The listing builds one solid part. Answer for the finished solid, in the listing's coordinates (mm). Face numbers are marked on the shaded views. A direction names the side the tool comes from. Give positions to 0.01 mm unless a question says otherwise; leave off trailing zeros. Loops run counter-clockwise (first coordinate to the right, second up) from the corner with the lowest first, then second, coordinate; pieces in that order, holes last. Notation, with made-up numbers: (-14, 51) - (14, 51) arc R4 cw to (14, 56) - close; hole circle Ø7 at (1, 0.5). An arc over 180 degrees is marked (long way). Write each question's results on one line, items separated by ' | '.
Autodesk Inventor part; units mm, degrees
ref_plane "YZ Plane" through (0, 0, 0) normal (1, 0, 0) x (0, 1, 0)
ref_plane "XZ Plane" through (0, 0, 0) normal (0, 1, 0) x (-1, 0, 0)
ref_plane "XY Plane" through (0, 0, 0) normal (0, 0, 1) x (1, 0, 0)
sketch "Sketch1" plane through (0, 0, 0) normal (1, 0, 0) x (0, 1, 0)
  line L0 (0, 0) -> (230.2002, 0)
  line L1 (230.2002, 0) -> (230.2002, -138.176)
  line L2 (230.2002, -138.176) -> (0, -138.176)
  line L3 (0, -138.176) -> (0, 0)
  dimension "d0" = 230.2002
  dimension "d1" = 138.176
extrude "Extrusion1" add sketch "Sketch1" along normal blind 266.7
sketch "Sketch2" plane through (266.7, 0, 0) normal (1, 0, 0) x (0, 0, -1)
  line L0 (0, 230.2002) -> (0, 0)
  line L1 (0, 0) -> (138.176, 0)
  line L2 (138.176, 0) -> (138.176, 230.2002)
  line L3 (138.176, 230.2002) -> (0, 230.2002)
  line L4 (19.05, 211.1502) -> (63.5, 211.1502)
  line L5 (63.5, 211.1502) -> (63.5, 19.05)
  line L6 (63.5, 19.05) -> (19.05, 19.05)
  line L7 (19.05, 19.05) -> (19.05, 211.1502)
  dimension "d4" = 19.05
  dimension "d5" = 63.5
  dimension "d7" = 19.05
  dimension "d17" = 19.05
extrude "Extrusion2" cut sketch "Sketch2" against normal blind 266.7 contours L4 L5 L6 L7
sketch "Sketch3" plane through (0, 0, 0) normal (-1, 0, 0) x (0, 0, 1)
  line L0 (-19.05, 211.1502) -> (-19.05, 19.05)
  line L1 (-19.05, 19.05) -> (-63.5, 19.05)
  line L2 (-63.5, 19.05) -> (-63.5, 211.1502)
  line L3 (-63.5, 211.1502) -> (-19.05, 211.1502)
  line L4 (0, 0) -> (0, 230.2002)
  line L5 (0, 230.2002) -> (-138.176, 230.2002)
  line L6 (-138.176, 230.2002) -> (-138.176, 0)
  line L7 (-138.176, 0) -> (0, 0)
  line L8 (-138.176, 103.2002) -> (-239.776, 103.2002)
  line L9 (-239.776, 103.2002) -> (-239.776, 141.3002)
  line L10 (-239.776, 141.3002) -> (-138.176, 141.3002)
  line L11 (-138.176, 141.3002) -> (-138.176, 103.2002)
  dimension "d11" = 101.6
  dimension "d12" = 38.1
  dimension "d14" = 127
extrude "Extrusion3" add sketch "Sketch3" against normal blind 63.5 contours L8 L9 L10 L6
properties part number "ShooterProto"
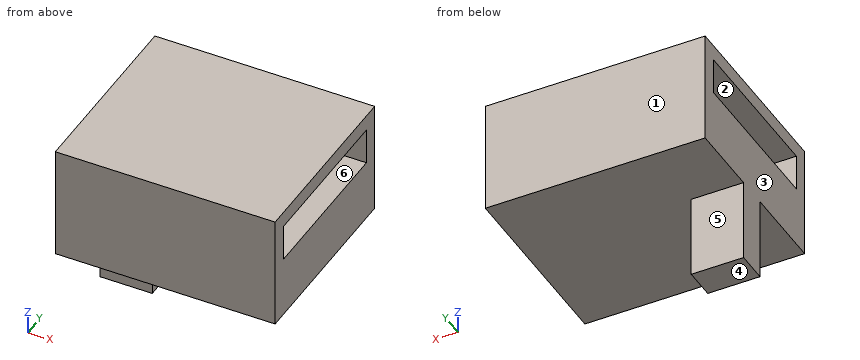
Item 1: A cutting plane is placed at C-C, the plane x = 35.5. Determine the outline of the cut face in (y, z).
Values found:
outline: (0, -138.18) - (103.2, -138.18) - (103.2, -239.78) - (141.3, -239.78) - (141.3, -138.18) - (230.2, -138.18) - (230.2, 0) - (0, 0) - close; hole (19.05, -63.5) - (211.15, -63.5) - (211.15, -19.05) - (19.05, -19.05) - close
Item 2: For a pull along Y with two mould halves and no side action, classify the marked faces 1, 2 and 3 as released by +Y, released by -Y, zero draft, split by the parting line, or undercut.
Values found:
face 1: released by +Y | face 2: undercut | face 3: zero draft
Item 3: A cutting plane is placed at B-B, the plane y = 94. Determine the outline of the cut face in (x, z).
Values found:
outline: (0, -138.18) - (266.7, -138.18) - (266.7, -63.5) - (0, -63.5) - close; (0, -19.05) - (266.7, -19.05) - (266.7, 0) - (0, 0) - close
Item 4: Flat-ended cylindrical pins translate along their axes: P1, Ø8, axis at x = 237, y = 173, coming from the +Z side; P2, Ø12, axis at x = 77, z = -145.5, coming from the -Y side; P3, Ø2, axis at x = 46, z = -204, coming from the -Y side; P4, Ø2, axis at x = 86.5, y = 160, coming from the -Z side. Find the tip coordinate at first contact, or state that the pin passes through.
Values found:
P1: stops at z = 0 | P2: passes through | P3: stops at y = 103.2 | P4: stops at z = -138.18
Item 5: Find the intervals of material crossed by line 1 along Z through (x, y) = (169, 205); line 2 along Y through (x, z) = (43, -30); line 3 along Y through (x, z) = (36, -169), in increasing order. Write a range as [from, to].
Values found:
line 1: z = [-138.18, -63.5], [-19.05, 0] | line 2: y = [0, 19.05], [211.15, 230.2] | line 3: y = [103.2, 141.3]
Item 6: A cutting plane is placed at D-D, the plane y = 130. Determine the outline of the cut face in (x, z), plus the area to 3 significant figures.
Values found:
outline: (0, -239.78) - (63.5, -239.78) - (63.5, -138.18) - (266.7, -138.18) - (266.7, -63.5) - (0, -63.5) - close; (0, -19.05) - (266.7, -19.05) - (266.7, 0) - (0, 0) - close | area: 31,400 mm²
Item 7: A cutting plane is placed at A-A, the plane z = -42.5. Determine the outline of the cut face in (x, y), plus the area to 3 significant figures.
Values found:
outline: (0, 0) - (266.7, 0) - (266.7, 19.05) - (0, 19.05) - close; (0, 211.15) - (266.7, 211.15) - (266.7, 230.2) - (0, 230.2) - close | area: 10,200 mm²
Item 8: For the marked faces 4, 5 and 6, determine the directions among +Z, -Z, +X, -X, +Y, -Y from which every point of the face is accessible in a straight line to the end or side of a thin tool.
Values found:
face 4: -Z, +X, -X, +Y, -Y | face 5: -Z, +X, -X, +Y | face 6: +X, -X
